Check sheet for the modelled part. Datum: model origin and axes. Units: mm. Face numbers are marked on the shaded views. A direction names the side the tool comes from. Round coordinates to 2 decimals unless told otherwise and drop trailing zeros. Loops run counter-clockwise (first coordinate to the right, second up) from the corner with the lowest first, then second, coordinate; pieces in that order, holes last. Notation, with made-up numbers: (54.5, 1) -> (60.5, 1) arc R12 cw to (60.5, 10) -> close; hole circle Ø10 at (84.25, 31.5). An arc over 180 degrees is marked (long way). Use one line per item in the form item = value. Start each with the question number.
(1) Go/stop test with flat-tipped pins: pin 1 (3 mm diameter, centred on x = 2.5, z = -1, fed in from +Y); pin 2 (3 mm diameter, centred on y = -10.5, z = -6, fed in from +X); pin 3 (5 mm diameter, centred on x = 12, z = 2.5, fed in from -Y). Record where each tip stops, or that it passes through.
(2) Sectioned sample at D-D (z = 1.75). Record the cut outline in (x, y).
(3) Set-up check for the marked faces 1 and 2: record each of +Z, -Z, +X, -X, +Y, -Y from which the full face is reachable in a straight line by a thin tool's end or side.
(4) Material ranges on probe 1 along Y at (x, z) = (0.5, -9); probe 2 along X at (y, z) = (2.5, 3); probe 3 along Y at (x, z) = (-12.5, -2.5), recorded low to high. Write a range as [from, to].
(5) Sectioned sample at C-C (y = -6.75). Record the cut outline in (x, z), and give its area (3 significant figures).
(6) Sectioned sample at B-B (z = -8.5). Record the cut outline in (x, y).
(7) Sectioned sample at A-A (x = 0). Record the cut outline in (y, z).
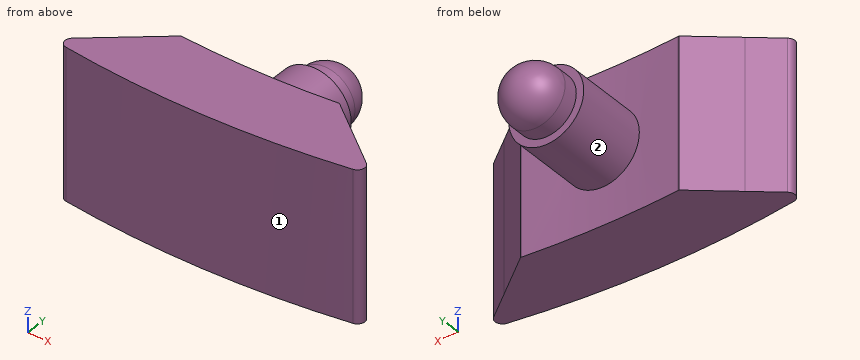
from build123d import *

# Parameters (mm, degrees)
F0_R          = 5
F1_DEPTH      = 10
F2_R          = 4
F3_DEPTH      = 6
F4_R          = 4
F6_DEPTH      = 10
F6_DEPTH_BACK = 10
F7_T4_DEPTH   = 20
F7_S5_R       = 120
F7_T6_DEPTH   = 12
F7_T10_DEPTH  = 20
F7_S11_R      = 120
F7_T12_DEPTH  = 12
F9_DEPTH      = 25
F10_R         = 1


# Not quite as in the source:
# - a fillet or chamfer that OpenCascade refuses, or shapes differently, is made with other operations: its cross-section is extruded or revolved along the edge and cut away or added


with BuildPart() as f1:
    # F0 (on Front) → F1 (new body)
    with BuildSketch(Plane.XZ):
        Circle(F0_R)
    extrude(amount=F1_DEPTH)

    # F2 (on face) → F3 (join)
    with BuildSketch(Plane(origin=(0, 0, 0), x_dir=(-1, 0, 0), z_dir=(0, 1, 0))):
        Circle(F2_R)
    extrude(amount=F3_DEPTH)

    # F4
    f4_edges = [f1.edges().sort_by_distance(p)[0] for p in [
        (4, 6, 0),
    ]]
    fillet(f4_edges, radius=F4_R)

    # F5 (on Top) → F6 (join, two sides)
    with BuildSketch(Plane.XY) as f6_sk:
        with BuildLine():
            ThreePointArc((10.4586891297, -9.543363771), (0, -10), (-10.4586891297, -9.543363771))
            Line((-10.4586891297, -9.543363771), (-10.8944678435, -14.5243372615))
            ThreePointArc((-10.8944678435, -14.5243372615), (-16.3157740275, -13.9306076717), (-21.7060222084, -13.1009691265))
            Line((-21.7060222084, -13.1009691265), (-22.5742630967, -18.0250078916))
            ThreePointArc((-22.5742630967, -18.0250078916), (0, -20), (22.5742630967, -18.0250078916))
            Line((22.5742630967, -18.0250078916), (21.7060222084, -13.1009691265))
            ThreePointArc((21.7060222084, -13.1009691265), (16.3157740275, -13.9306076717), (10.8944678435, -14.5243372615))
            Line((10.8944678435, -14.5243372615), (10.4586891297, -9.543363771))
        make_face()
    extrude(amount=F6_DEPTH)
    extrude(f6_sk.sketch, amount=-F6_DEPTH_BACK)

    # F7: chamfer of 5 on 2 edges, made by hand


with BuildPart() as f7_tool2:
    # F7_s3 → F7_t4 (new body)
    with BuildSketch(Plane.XY.offset(-10)):
        with BuildLine():
            Line((-16.0735207845, -13.962260102), (-10.4496064627, -9.4395484116))
            Line((-10.4496064627, -9.4395484116), (-10.8944678435, -14.5243372615))
            ThreePointArc((-10.8944678435, -14.5243372615), (-13.5571939783, -14.262635138), (-16.0735207845, -13.962260102))
        make_face()
    extrude(amount=F7_T4_DEPTH)

    # F7_s5 → F7_t6 (cut, symmetric)
    with BuildSketch(Plane.XY):
        with Locations((0, 110)):
            Circle(F7_S5_R)
    extrude(amount=F7_T6_DEPTH, both=True, mode=Mode.SUBTRACT)


with BuildPart() as f1_1:
    add(f1.part)

    # F7_t1: union F7_tool2
    add(f7_tool2.part)


with BuildPart() as f7_tool8:
    # F7_s9 → F7_t10 (new body)
    with BuildSketch(Plane.XY.offset(10)):
        with BuildLine():
            Line((10.4496064627, -9.4395484116), (16.0735207845, -13.962260102))
            ThreePointArc((16.0735207845, -13.962260102), (13.5571939783, -14.262635138), (10.8944678435, -14.5243372615))
            Line((10.8944678435, -14.5243372615), (10.4496064627, -9.4395484116))
        make_face()
    extrude(amount=-F7_T10_DEPTH)

    # F7_s11 → F7_t12 (cut, symmetric)
    with BuildSketch(Plane.XY):
        with Locations((0, 110)):
            Circle(F7_S11_R)
    extrude(amount=F7_T12_DEPTH, both=True, mode=Mode.SUBTRACT)


with BuildPart() as f1_2:
    add(f1_1.part)

    # F7_t7: union F7_tool8
    add(f7_tool8.part)

    # F8 (on face) → F9 (cut)
    with BuildSketch(Plane.XY.offset(10)):
        Polygon((-22.1401426525, -18.8409940359), (-16.0735207845, -13.962260102), (-26.2115597725, -8.7402015924), (-26.2115597725, -18.8409940359), align=None)
        Polygon((26.2115597725, -8.7402015924), (16.0735207845, -13.962260102), (22.1401426525, -18.8409940359), (26.2115597725, -18.8409940359), align=None)
    extrude(amount=-F9_DEPTH, mode=Mode.SUBTRACT)

    # F10
    f10_edges = [f1_2.edges().sort_by_distance(p)[0] for p in [
        (-21.380167, -18.229827, 0),
        (21.380167, -18.229827, 0),
    ]]
    fillet(f10_edges, radius=F10_R)


solid = f1_2.part
Checks:
q1.pin_1 = 5.82
q1.pin_2 = 13.63
q1.pin_3 = -19.65
q2.outline = (-19.62, -16.81) arc R1 ccw to (-19.14, -18.58) arc R130 ccw to (19.14, -18.58) arc R1 ccw to (19.62, -16.81) -> (10.57, -9.53) arc R120 cw to (4.68, -9.91) -> (4.68, 0) -> (3.6, 0) -> (3.6, 2) arc R3.6 ccw to (-3.6, 2) -> (-3.6, 0) -> (-4.68, 0) -> (-4.68, -9.91) arc R120 cw to (-10.57, -9.53) -> close
q3.face_1 = +Z, -Z, -Y
q3.face_2 = +Y
q4.probe_1 = [-20, -10]
q4.probe_2 = [-2.6, 2.6]
q4.probe_3 = [-19.4, -11.09]
q5.outline = circle Ø10 at (0, 0)
q5.area = 78.5 mm2
q6.outline = (-19.62, -16.81) arc R1 ccw to (-19.14, -18.58) arc R130 ccw to (19.14, -18.58) arc R1 ccw to (19.62, -16.81) -> (10.57, -9.53) arc R120 cw to (-10.57, -9.53) -> close
q7.outline = (-20, -10) -> (-10, -10) -> (-10, -5) -> (0, -5) -> (0, -4) -> (2, -4) arc R4 ccw to (2, 4) -> (0, 4) -> (0, 5) -> (-10, 5) -> (-10, 10) -> (-20, 10) -> close
